from build123d import *

# Parameters (mm, degrees)
SKETCH1_W                       = 44
SKETCH1_H                       = 162.947999986
EXTRUDE1_DEPTH                  = 9.525
SKETCH5_W                       = 44
SKETCH5_H                       = 104.527999986
EXTRUDE3_DEPTH                  = 2
SKETCH7_W                       = 44
SKETCH7_H                       = 25.735194666
EXTRUDE5_DEPTH                  = 5.25
SKETCH6_W                       = 44
SKETCH6_H                       = 31.986263093
EXTRUDE4_DEPTH                  = 4.032
F_1_4_0_25_DIAMETER_HOLE1_D     = 6.35
F_1_4_0_25_DIAMETER_HOLE1_DEPTH = 18.618
SKETCH8_W                       = 44
SKETCH8_H                       = 6.307
EXTRUDE6_DEPTH                  = 50.8
CBORE_FOR_M3_SBHCS1_D           = 3.6
CBORE_FOR_M3_SBHCS1_CBORE_D     = 6.7
CBORE_FOR_M3_SBHCS1_CBORE_DEPTH = 1.65
SKETCH12_R                      = 1.190625
CUT_EXTRUDE1_DEPTH              = 135.28690768
M4_CLEARANCE_HOLE1_D            = 4.5
M4_CLEARANCE_HOLE1_DEPTH        = 8.204
CHAMFER1_SIZE                   = 3


with BuildPart() as part:
    # Sketch1 → Extrude1 (new body)
    with BuildSketch(Plane(origin=(0, 0, 0), x_dir=(1, 0, 0), z_dir=(0, 1, 0))):
        Rectangle(SKETCH1_W, SKETCH1_H)
    extrude(amount=EXTRUDE1_DEPTH)

    # Sketch5 → Extrude3 (cut)
    with BuildSketch(Plane(origin=(0, 9.525, 0), x_dir=(1, 0, 0), z_dir=(0, 1, 0))):
        with Locations((0, 29.21)):
            Rectangle(SKETCH5_W, SKETCH5_H)
    extrude(amount=-EXTRUDE3_DEPTH, mode=Mode.SUBTRACT)

    # Sketch7 → Extrude5 (cut)
    with BuildSketch(Plane(origin=(0, 7.525, 0), x_dir=(1, 0, 0), z_dir=(0, 1, 0))):
        with Locations((0, 68.60640266)):
            Rectangle(SKETCH7_W, SKETCH7_H)
    extrude(amount=-EXTRUDE5_DEPTH, mode=Mode.SUBTRACT)

    # Sketch6 → Extrude4 (add)
    with BuildSketch(Plane.XZ):
        with Locations((0, -65.480868447)):
            Rectangle(SKETCH6_W, SKETCH6_H)
    extrude(amount=EXTRUDE4_DEPTH)

    # 1/4 (0.25) Diameter Hole1
    with Locations(Plane(origin=(-11.909442165, -4.032, 7.994157722), x_dir=(1, 0, 0), z_dir=(0, -1, 0))):
        with Locations((11.909442165, -70.418157729)):
            Hole(F_1_4_0_25_DIAMETER_HOLE1_D / 2, depth=F_1_4_0_25_DIAMETER_HOLE1_DEPTH)

    # Sketch8 → Extrude6 (add)
    with BuildSketch(Plane(origin=(0, 0, -81.473999993), x_dir=(-1, 0, 0), z_dir=(0, 0, -1))):
        with Locations((0, -0.8785)):
            Rectangle(SKETCH8_W, SKETCH8_H)
    extrude(amount=EXTRUDE6_DEPTH)

    # CBORE for M3 SBHCS1 (through all)
    with Locations(Plane.XZ):
        with Locations((-13, 77.473999993), (13, 77.473999993), (13, 27.473999993), (-13, 27.473999993)):
            CounterBoreHole(CBORE_FOR_M3_SBHCS1_D / 2, CBORE_FOR_M3_SBHCS1_CBORE_D / 2, CBORE_FOR_M3_SBHCS1_CBORE_DEPTH)

    # Sketch12 → Cut-Extrude1 (cut, through all)
    with BuildSketch(Plane(origin=(0, 2.275, 0), x_dir=(-1, 0, 0), z_dir=(0, 1, 0))):
        with Locations(Location((0.10007052, -127.574998873, 0), (0, 0, 90))):
            Circle(SKETCH12_R)
        with Locations(Location((0.10007052, -107.254998873, 0), (0, 0, 90))):
            Circle(SKETCH12_R)
    extrude(amount=-CUT_EXTRUDE1_DEPTH, mode=Mode.SUBTRACT)

    # M4 Clearance Hole1
    with Locations(Plane(origin=(0, 2.275, 0), x_dir=(-1, 0, 0), z_dir=(0, 1, 0))):
        with Locations((0.10007052, -117.540271762)):
            Hole(M4_CLEARANCE_HOLE1_D / 2, depth=M4_CLEARANCE_HOLE1_DEPTH)

    # Chamfer1
    chamfer1_edges = [part.edges().sort_by_distance(p)[0] for p in [
        (-2.35007052, 2.275, -117.540271762),
    ]]
    chamfer(chamfer1_edges, length=CHAMFER1_SIZE)


solid = part.part
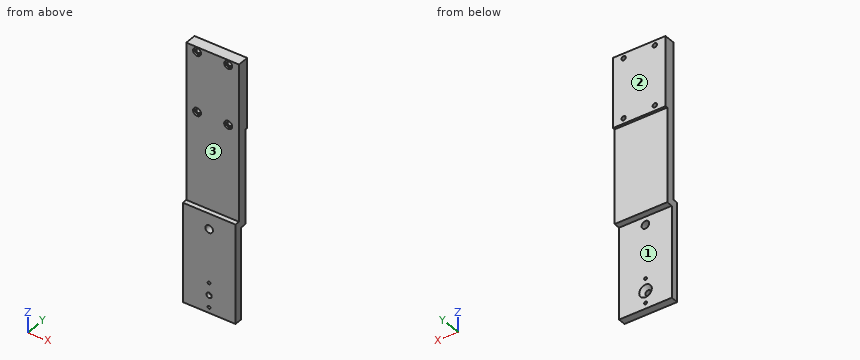
Can you work these out from the model? Positions are in its coordinate system, mm. Face numbers are marked on the shaded views. A direction names the side the tool comes from. Coordinates: 2 decimals unless noted, no trailing zeros. Write each loop counter-clockwise with the first axis right and the second up, starting at its lowest first coordinate (ties: lowest second). Pieces come first, ordered by that corner, then holes. Notation, with made-up numbers: (48.25, 44) -> (91.25, 44) arc R19 cw to (91.25, 53) -> close; hole circle Ø9 at (-14, 38). An arc over 180 degrees is marked (long way). Write item = value, one per line.
(1) Imagine slicing it at A-A (x = 13). Please give me the cut outline in (y, z) (3 decimals), and give its area (3 significant figures).
Verdict:
outline = (-4.032, -132.274) -> (2.275, -132.274) -> (2.275, -55.739) -> (7.525, -55.739) -> (7.525, 23.054) -> (9.525, 23.054) -> (9.525, 25.674) -> (1.65, 25.674) -> (1.65, 24.124) -> (0, 24.124) -> (0, -49.488) -> (-4.032, -49.488) -> close; (0, 30.824) -> (1.65, 30.824) -> (1.65, 29.274) -> (9.525, 29.274) -> (9.525, 75.674) -> (1.65, 75.674) -> (1.65, 74.124) -> (0, 74.124) -> close; (0, 80.824) -> (1.65, 80.824) -> (1.65, 79.274) -> (9.525, 79.274) -> (9.525, 81.474) -> (0, 81.474) -> close
area = 1,580 mm^2
(2) Imagine slicing it at B-B (z = 16). Please give me the cut outline in (x, y) (3 decimals).
Verdict:
outline = (-22, 0) -> (22, 0) -> (22, 7.525) -> (-22, 7.525) -> close
(3) If I drill on probe 1 along Z at (x, y) = (-13, 7.25); probe 2 along Z at (x, y) = (-2, -2.75); probe 3 along Y at (x, z) = (17.5, -98) (3 decimals), over which ranges is the centre line in solid material (lowest first)?
Verdict:
probe_1 = -55.74 to 25.67, 29.27 to 75.67, 79.27 to 81.47
probe_2 = -132.27 to -118.75, -116.33 to -64.89, -59.96 to -49.49
probe_3 = -4.032 to 2.275
(4) On a 3-axis mill with a long thin cutter (end or side, diameter ignored), from which of +Z, -Z, +X, -X, +Y, -Y can I reach the whole of each face in a straight line? I mean the marked faces 1, 2 and 3. Say none if no direction works.
Verdict:
face_1 = -Z, +X, -X, +Y
face_2 = +Z, -Z, +X, -X, +Y
face_3 = +Z, +X, -X, -Y
(5) For pin 1 (2 mm diameter, centred on x = -6.5, y = 9, fed in from -Z); pin 2 (8 mm diameter, centred on x = -16, z = 52, fed in from -Y); pin 3 (6 mm diameter, centred on x = -0.1, z = -117.54, fed in from +Y); pin 4 (3 mm diameter, centred on y = -2, z = -0.5, fed in from +X), each with a flat end and sliding along its axis, tell me the tip position at first contact or that it passes through.
Verdict:
pin_1 = 23.05
pin_2 = 0
pin_3 = 0.03
pin_4 = through
